Autodesk Inventor part; units mm, degrees
ref_plane "YZ Plane" through (0, 0, 0) normal (1, 0, 0) x (0, 1, 0)
ref_plane "XY Plane" through (0, 0, 0) normal (0, 0, 1) x (1, 0, 0)
sketch "Sketch1" plane through (0, 0, 0) normal (1, 0, 0) x (0, 1, 0)
  circle A0 centre (0, 0) radius 10.5
  dimension "d0" = 21
extrude "Extrusion1" add sketch "Sketch1" along normal blind 227
sketch "Sketch2" plane through (227, 0, 0) normal (1, 0, 0) x (0, 0, -1)
  circle A0 centre (0, 0) radius 3
  dimension "d3" = 6
sketch "Sketch3" plane through (0, 0, 0) normal (-1, 0, 0) x (0, 0, 1)
  circle A0 centre (0, 0) radius 3
  dimension "d4" = 6
extrude "Extrusion2" add sketch "Sketch3" along normal blind 8
extrude "Extrusion3" add sketch "Sketch2" along normal blind 28
sketch "Sketch4" plane through (-8, 0, 0) normal (-1, 0, 0) x (0, 0, 1)
  circle A0 centre (0, 0) radius 2.5
  dimension "d9" = 5
extrude "Extrusion4" add sketch "Sketch4" along normal blind 11
ref_plane "Work Plane1" through (-8, 2.5, 0) normal (0, 1, 0) x (-1, 0, 0)
sketch "Sketch5" plane through (-8, 2.5, 0) normal (0, 1, 0) x (-1, 0, 0)
  circle A0 centre (4, 0) radius 1
  line L0 (0, -3) -> (0, 3)
  point P0 (-8, 0)
  dimension "d12" = 2
  dimension "d13" = 4
extrude "Extrusion5" add sketch "Sketch5" along normal blind 3.5 and the other way blind 8.5
sketch "Sketch6" plane through (-19, 0, 0) normal (-1, 0, 0) x (0, 0, 1)
  circle A0 centre (0, 0) radius 2
  dimension "d16" = 4
extrude "Extrusion6" add sketch "Sketch6" along normal blind 11
properties part number "RouleauFriction"
The listing builds one solid part. Answer for the finished solid, in the listing's coordinates (mm). A direction names the side the tool comes from. Round coordinates to 2 decimals unless told otherwise and drop trailing zeros. Loops run counter-clockwise (first coordinate to the right, second up) from the corner with the lowest first, then second, coordinate; pieces in that order, holes last.
1) A cutting plane is placed at D-D on z = 7.25. Determine the outline of the cut face in (x, y), plus the area to 3 significant figures.
Outcome:
outline: (0, -7.6) - (227, -7.6) - (227, 7.6) - (0, 7.6) - close
area: 3,450 mm2
2) For a pull along X with two mould halves and no side action, classify faces 4 (the face through (-19, 2, -1)), 5 (the face through (-8, 2, -2)), 6 (the face through (111.9, 10, -3.2)) as released by +X, released by -X, zero draft, split by the parting line, or undercut.
Outcome:
face 4: released by -X
face 5: undercut
face 6: zero draft
3) A cutting plane is placed at A-A on x = 235. Determine the outline of the cut face in (y, z).
Outcome:
outline: circle Ø6 at (0, 0)
4) A cutting plane is placed at B-B on z = -8. Determine the outline of the cut face in (x, y), plus the area to 3 significant figures.
Outcome:
outline: (0, -6.8) - (227, -6.8) - (227, 6.8) - (0, 6.8) - close
area: 3,090 mm2
5) Consider line 1 (X direction, y = 8.5, z = -1.75); line 2 (X direction, y = -4.75, z = -0.75); line 3 (X direction, y = -2.25, z = 1). Determine where each line is inside the solid, lowest interval first.
Outcome:
line 1: x = 0 to 227
line 2: x = -12.66 to -11.34, 0 to 227
line 3: x = -19 to 255
6) Given P1, Ø1, axis at x = 104, z = -6.5, coming from the -Y side; P2, Ø1.6, axis at x = -11.5, z = 0, coming from the -Y side; P3, Ø1.5, axis at x = 124.5, z = -5, coming from the -Y side, each flat-ended and moving along its own axis, determine where each tip first touches the part or whether it passes through.
Outcome:
P1: stops at y = -8.62
P2: stops at y = -6
P3: stops at y = -9.6
7) A cutting plane is placed at C-C on x = 50. Determine the outline of the cut face in (y, z).
Outcome:
outline: circle Ø21 at (0, 0)
8) For faces 1 (the face through (227, 2.2, 2.5)), 2 (the face through (-4, 0, -3)), 3 (the face through (255, 0, 0)), determine the directions among +Z, -Z, +X, -X, +Y, -Y from which every point of the face is accessible in a straight line to the end or side of a thin tool.
Outcome:
face 1: +X
face 2: none
face 3: +Z, -Z, +X, +Y, -Y
